```python
from build123d import *

# Parameters (mm, degrees)
F0_W      = 1524
F0_H      = 914.4
F1_DEPTH  = 457.2
F2_W      = 736.6
F2_H      = 736.6
F3_DEPTH  = 2133.6
F4_W      = 1447.8
F4_H      = 838.2
F4_W_2    = 533.4
F4_H_2    = 1529.586154
F5_DEPTH  = 914.4
F6_W      = 736.6
F6_H      = 602.486154
F7_DEPTH  = 609.6
F8_W      = 1485.9
F8_H      = 736.6
F9_DEPTH  = 914.4
F10_DEPTH = 914.4
F11_W     = 533.4
F11_H     = 736.6
F12_DEPTH = 1605.786154


with BuildPart() as f1:
    # F0 (on Front) → F1 (new body, symmetric)
    with BuildSketch(Plane.XZ):
        Rectangle(F0_W, F0_H)
        Polygon((762, 1148.586154), (762, 457.2), (762, -457.2), (1371.6, -457.2), (1371.6, 1148.586154), align=None)
    extrude(amount=F1_DEPTH, both=True)

    # F2 (on face) → F3 (cut, through all)
    with BuildSketch(Plane(origin=(-762, 0, 0), x_dir=(0, -1, 0), z_dir=(-1, 0, 0))):
        Rectangle(F2_W, F2_H)
    extrude(amount=-F3_DEPTH, mode=Mode.SUBTRACT)

    # F4 (on face) → F5 (cut, through all)
    with BuildSketch(Plane.XZ.offset(457.2)):
        Rectangle(F4_W, F4_H)
        with Locations((1066.8, 345.693077)):
            Rectangle(F4_W_2, F4_H_2)
    extrude(amount=-F5_DEPTH, mode=Mode.SUBTRACT)

    # F6 (on face) → F7 (cut, through all)
    with BuildSketch(Plane(origin=(762, 0, 0), x_dir=(0, -1, 0), z_dir=(-1, 0, 0))):
        with Locations((0, 758.443077)):
            Rectangle(F6_W, F6_H)
    extrude(amount=-F7_DEPTH, mode=Mode.SUBTRACT)

    # F8 (on face) → F9 (cut, through all)
    with BuildSketch(Plane.XY.offset(457.2)):
        with Locations((19.05, 0)):
            Rectangle(F8_W, F8_H)
    extrude(amount=-F9_DEPTH, mode=Mode.SUBTRACT)

    # F8 (on face) → F10 (cut, through all)
    with BuildSketch(Plane.XY.offset(457.2)):
        with Locations((19.05, 0)):
            Rectangle(F8_W, F8_H)
    extrude(amount=-F10_DEPTH, mode=Mode.SUBTRACT)

    # F11 (on face) → F12 (cut, through all)
    with BuildSketch(Plane(origin=(0, 0, -457.2), x_dir=(1, 0, 0), z_dir=(0, 0, -1))):
        with Locations((1066.8, 0)):
            Rectangle(F11_W, F11_H)
    extrude(amount=-F12_DEPTH, mode=Mode.SUBTRACT)


solid = f1.part
```
For this review, take the finished solid that the model builds, in its own axes (mm). A direction names the side the tool comes from. Coordinates: 2 decimals unless noted, no trailing zeros. Order: outer loops, then holes, each group sorted by start corner. A loop starts at its lowest first (then second) coordinate and runs counter-clockwise, first axis right, second up. Notation, with made-up numbers: (37, 58) - (82, 58) arc R22 ccw to (82, 71) - close; hole circle Ø10 at (-12, 32). An arc over 180 degrees is marked (long way). Answer as a JSON object with one key per item and string values. Group by question number.
1. We need section B-B on x = 1170.5. State the section outline as (y, z) points, then the cut area to 3 significant figures.
2. For faces 4 (the flat face through (-10, -413, -419.1)), 5 (the flat face through (762, -5, 413)), 6 (the flat face through (762, 32, 1061)), 7 (the flat face through (204, -368.3, 442)), list the 3-axis set-ups (+Z, -Z, +X, -X, +Y, -Y) from which the entire face can be reached by the end or side of a thin tool; tool diameter is ignored.
3. We need section A-A on z = 272. State the section outline as (x, y) points, then the cut area to 3 significant figures.
4. Clearance check with a flat-ended pin moving along its axis: P1, Ø11.5, axis at x = -735, y = -81, coming from the +Z side. State where the tip first meets the part, or that it passes through.
5. We need section C-C on y = 101. Give the number of separate pieces and of enclosed holes in the cut face, then the cut area to 3 significant figures.
6. The part is to be moulded in two halves that separate along X. For faces 1 (the flat face through (723.9, 412, -6)), 2 (the flat face through (-762, -6, -413)), 3 (the flat face through (221, 370, -457.2)), say which applies: pulls with the +X half, pulls with the -X half, needs draft (parallel to the pull), parting line crosses it, or undercut.
7. We need section D-D on z = 815.5. State the section outline as (x, y) points, then the cut area to 3 significant figures.
8. For probe 1 along X at (y, z) = (-25, 416.5); probe 2 along Y at (x, z) = (734.5, -18.5); probe 3 along Z at (x, y) = (614, 401), list the stretches that pass through material, from the lowest coordinate up.
Final values:
{
 "1": {"outline": "(-457.2, -457.2) - (-368.3, -457.2) - (-368.3, -419.1) - (-457.2, -419.1) - close; (-457.2, 1110.49) - (-368.3, 1110.49) - (-368.3, 1148.59) - (-457.2, 1148.59) - close; (368.3, -457.2) - (457.2, -457.2) - (457.2, -419.1) - (368.3, -419.1) - close; (368.3, 1110.49) - (457.2, 1110.49) - (457.2, 1148.59) - (368.3, 1148.59) - close", "area": "13,500 mm²"},
 "2": {"face 4": "+Y, -Y", "face 5": "+Z, -Z", "face 6": "+Z, -X, +Y, -Y", "face 7": "none"},
 "3": {"outline": "(-762, -457.2) - (-723.9, -457.2) - (-723.9, -368.3) - (-762, -368.3) - close; (-762, 368.3) - (-723.9, 368.3) - (-723.9, 457.2) - (-762, 457.2) - close; (723.9, -457.2) - (800.1, -457.2) - (800.1, -368.3) - (723.9, -368.3) - close; (723.9, 368.3) - (800.1, 368.3) - (800.1, 457.2) - (723.9, 457.2) - close; (1333.5, -457.2) - (1371.6, -457.2) - (1371.6, -368.3) - (1333.5, -368.3) - close; (1333.5, 368.3) - (1371.6, 368.3) - (1371.6, 457.2) - (1333.5, 457.2) - close", "area": "27,100 mm²"},
 "4": {"P1": "z = 457.2"},
 "5": {"separate pieces": "8", "enclosed holes": "0", "area": "27,100 mm²"},
 "6": {"face 1": "undercut", "face 2": "pulls with the -X half", "face 3": "needs draft"},
 "7": {"outline": "(762, -457.2) - (800.1, -457.2) - (800.1, -368.3) - (762, -368.3) - close; (762, 368.3) - (800.1, 368.3) - (800.1, 457.2) - (762, 457.2) - close; (1333.5, -457.2) - (1371.6, -457.2) - (1371.6, -368.3) - (1333.5, -368.3) - close; (1333.5, 368.3) - (1371.6, 368.3) - (1371.6, 457.2) - (1333.5, 457.2) - close", "area": "13,500 mm²"},
 "8": {"probe 1": "-762 to -723.9, 762 to 800.1, 1333.5 to 1371.6", "probe 2": "-457.2 to -368.3, 368.3 to 457.2", "probe 3": "-457.2 to -419.1, 419.1 to 457.2"}
}
